from build123d import *

# Parameters (mm, degrees)
SKETCH10_R              = 10
BOSS_EXTRUDE1_DEPTH     = 5
CUT_EXTRUDE3_DEPTH      = 45
CUT_EXTRUDE3_DEPTH_BACK = 20
CUT_EXTRUDE5_DEPTH      = 5
BOSS_EXTRUDE2_DEPTH     = 5
SKETCH14_R              = 1
BOSS_EXTRUDE3_DEPTH     = 3
BOSS_EXTRUDE4_START     = 3
SKETCH15_R              = 1
BOSS_EXTRUDE4_DEPTH     = 3
CUT_EXTRUDE6_DEPTH      = 10
CUT_EXTRUDE6_DRAFT      = -10
SKETCH18_W              = 50.237541655
SKETCH18_H              = 20.454146011
CUT_EXTRUDE7_DEPTH      = 7
CUT_EXTRUDE7_DRAFT      = -30


with BuildPart() as part:
    # Sketch1 → Revolve1 (revolve)
    with BuildSketch(Plane.XY, mode=Mode.PRIVATE) as revolve1_sk:
        with BuildLine():
            Line((20.9, 0), (23.871591838, 0))
            Line((23.871591838, 0), (23.871591838, 4))
            Line((23.871591838, 4), (22.9, 4.236662843))
            Line((22.9, 4.236662843), (22.9, 11.874576818))
            ThreePointArc((22.9, 11.874576818), (23.83692213, 16.100759435), (26.472123903, 19.535021249))
            Line((26.472123903, 19.535021249), (26.427876097, 19.497892931))
            ThreePointArc((26.427876097, 19.497892931), (29.06307787, 22.932154745), (30, 27.158337362))
            Line((30, 27.158337362), (30, 50))
            ThreePointArc((30, 50), (28.828427125, 52.828427125), (26, 54))
            Line((26, 54), (0, 54))
            Line((0, 54), (0, 15))
            Line((0, 15), (19.9, 15))
            ThreePointArc((19.9, 15), (20.607106781, 14.707106781), (20.9, 14))
            Line((20.9, 14), (20.9, 0))
        make_face()
    revolve(revolve1_sk.sketch.rotate(Axis((0, 0, 0), (0, 1, 0)), 90), axis=Axis((0, 0, 0), (0, 1, 0)))

    # Sketch10 → Boss-Extrude1 (add)
    with BuildSketch(Plane(origin=(0, 0, -30), x_dir=(-1, 0, 0), z_dir=(0, 0, -1))):
        with Locations((3.346345887, 38.658337362)):
            Circle(SKETCH10_R)
    extrude(amount=-BOSS_EXTRUDE1_DEPTH)

    # Sketch11 → Cut-Extrude3 (cut, two sides: drawn at the far end of the back side and taken through both)
    with BuildSketch(Plane(origin=(0, 17, 0), x_dir=(1, 0, 0), z_dir=(0, 1, 0)).offset(-CUT_EXTRUDE3_DEPTH_BACK)):
        with BuildLine():
            Line((-17.5, 0), (17.5, 0))
            ThreePointArc((17.5, 0), (0, 17.5), (-17.5, 0))
        make_face()
    extrude(amount=CUT_EXTRUDE3_DEPTH + CUT_EXTRUDE3_DEPTH_BACK, mode=Mode.SUBTRACT)

    # Sketch9 → Cut-Extrude5 (cut)
    with BuildSketch(Plane(origin=(0, 54, 0), x_dir=(1, 0, 0), z_dir=(0, 1, 0))):
        with BuildLine():
            Line((-30, 0), (30, 0))
            ThreePointArc((30, 0), (0, 30), (-30, 0))
        make_face()
    extrude(amount=-CUT_EXTRUDE5_DEPTH, mode=Mode.SUBTRACT)

    # Sketch13 → Boss-Extrude2 (add)
    with BuildSketch(Plane(origin=(0, 0, 0), x_dir=(-1, 0, 0), z_dir=(0, 0, -1))):
        with BuildLine():
            Line((22.5, 53.5), (26.5, 53.5))
            ThreePointArc((26.5, 53.5), (26.853553391, 53.353553391), (27, 53))
            Line((27, 53), (27, 51))
            ThreePointArc((27, 51), (26.853553391, 50.646446609), (26.5, 50.5))
            Line((26.5, 50.5), (22.5, 50.5))
            ThreePointArc((22.5, 50.5), (22.146446609, 50.646446609), (22, 51))
            Line((22, 51), (22, 53))
            ThreePointArc((22, 53), (22.146446609, 53.353553391), (22.5, 53.5))
        make_face()
        with BuildLine():
            Line((-26.5, 53.5), (-22.5, 53.5))
            ThreePointArc((-22.5, 53.5), (-22.146446609, 53.353553391), (-22, 53))
            Line((-22, 53), (-22, 51))
            ThreePointArc((-22, 51), (-22.146446609, 50.646446609), (-22.5, 50.5))
            Line((-22.5, 50.5), (-26.5, 50.5))
            ThreePointArc((-26.5, 50.5), (-26.853553391, 50.646446609), (-27, 51))
            Line((-27, 51), (-27, 53))
            ThreePointArc((-27, 53), (-26.853553391, 53.353553391), (-26.5, 53.5))
        make_face()
    extrude(amount=BOSS_EXTRUDE2_DEPTH)

    # Sketch14 → Boss-Extrude3 (add)
    with BuildSketch(Plane.ZY.offset(-22)):
        with Locations(Location((-3, 52, 0), (0, 0, 270))):
            Circle(SKETCH14_R)
    extrude(amount=BOSS_EXTRUDE3_DEPTH)

    # Sketch15 → Boss-Extrude4 (add)
    with BuildSketch(Plane(origin=(-22, 0, 0), x_dir=(0, 0, -1), z_dir=(1, 0, 0)).offset(BOSS_EXTRUDE4_START)):
        with Locations(Location((3, 52, 0), (0, 0, 270))):
            Circle(SKETCH15_R)
    extrude(amount=-BOSS_EXTRUDE4_DEPTH)


with BuildPart() as cut_extrude6_tool:
    # Sketch17 → Cut-Extrude6 (with draft: the straight prism first)
    with BuildSketch(Plane(origin=(0, 0, 0), x_dir=(-1, 0, 0), z_dir=(0, 0, -1))):
        with BuildLine():
            ThreePointArc((-24.47851765, 47.302362136), (-25.892731213, 46.716575698), (-26.47851765, 45.302362136))
            Line((-26.47851765, 45.302362136), (-26.47851765, 25.01560965))
            ThreePointArc((-26.47851765, 25.01560965), (-25.892731213, 23.601396087), (-24.47851765, 23.01560965))
            Line((-24.47851765, 23.01560965), (25.354900287, 23.01560965))
            ThreePointArc((25.354900287, 23.01560965), (26.769113849, 23.601396087), (27.354900287, 25.01560965))
            Line((27.354900287, 25.01560965), (27.354900287, 45.302362136))
            ThreePointArc((27.354900287, 45.302362136), (26.769113849, 46.716575698), (25.354900287, 47.302362136))
            Line((25.354900287, 47.302362136), (-24.47851765, 47.302362136))
        make_face()
    extrude(amount=-CUT_EXTRUDE6_DEPTH)
    # Cut-Extrude6: the draft: its side faces are tilted about the plane it starts from
    cut_extrude6_sides = [cut_extrude6_tool.faces().sort_by_distance(p)[0] for p in [
        (25.892731213, 46.716575698, 5),
        (26.47851765, 35.158985893, 5),
        (25.892731213, 23.601396087, 5),
        (-0.438191318, 23.01560965, 5),
        (-26.769113849, 23.601396087, 5),
        (-27.354900287, 35.158985893, 5),
        (-26.769113849, 46.716575698, 5),
        (-0.438191318, 47.302362136, 5),
    ]]
    draft(cut_extrude6_sides, Plane(origin=(0, 0, 0), x_dir=(-1, 0, 0), z_dir=(0, 0, -1)), CUT_EXTRUDE6_DRAFT)


with BuildPart() as part_1:
    add(part.part)

    # Cut-Extrude6: cut by cut_extrude6_tool
    add(cut_extrude6_tool.part, mode=Mode.SUBTRACT)


with BuildPart() as cut_extrude7_tool:
    # Sketch18 → Cut-Extrude7 (with draft: the straight prism first)
    with BuildSketch(Plane(origin=(0, 0, 10), x_dir=(-1, 0, 0), z_dir=(0, 0, -1))):
        with Locations((0.403522985, 35.07528913)):
            Rectangle(SKETCH18_W, SKETCH18_H)
    extrude(amount=-CUT_EXTRUDE7_DEPTH)
    # Cut-Extrude7: the draft: its side faces are tilted about the plane it starts from
    cut_extrude7_sides = [cut_extrude7_tool.faces().sort_by_distance(p)[0] for p in [
        (24.715247843, 35.07528913, 13.5),
        (-0.403522984, 24.848216125, 13.5),
        (-25.522293812, 35.07528913, 13.5),
        (-0.403522984, 45.302362136, 13.5),
    ]]
    draft(cut_extrude7_sides, Plane(origin=(0, 0, 10), x_dir=(-1, 0, 0), z_dir=(0, 0, -1)), CUT_EXTRUDE7_DRAFT)


with BuildPart() as part_2:
    add(part_1.part)

    # Cut-Extrude7: cut by cut_extrude7_tool
    add(cut_extrude7_tool.part, mode=Mode.SUBTRACT)


solid = part_2.part
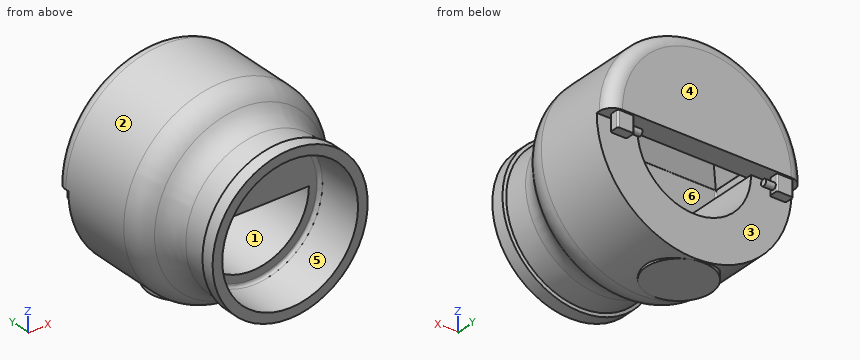
Geometry: final body of the model. Coordinates: model frame, mm. Face numbers are marked on the shaded views. A direction names the side the tool comes from. Round coordinates to 2 decimals unless told otherwise and drop trailing zeros. Loops run counter-clockwise (first coordinate to the right, second up) from the corner with the lowest first, then second, coordinate; pieces in that order, holes last. Notation, with made-up numbers: (36, 49.5) - (83, 49.5) arc R19 ccw to (83, 69.5) - close; hole circle Ø3 at (50, 1). An arc over 180 degrees is marked (long way). Write each question's results on one line, items separated by ' | '. Start each with the question number.
1) Mould query, pull axis X, two halves, no side actions, for the marked faces 1, 2 and 3. Classes: released by +X, released by -X, zero draft, split by the parting line, or undercut.
2) First-contact query: P1, Ø0.9, axis at x = -23.5, y = 52, coming from the -Z side; P2, Ø2, axis at y = 52, z = -1.5, coming from the -X side; P3, Ø1, axis at y = 52, z = -3.5, coming from the +X side. Flat tips, straight axial feed; report the tip coordinate or a pass-through.
3) Access query for the marked faces 4, 5 and 6. Directions: +Z, -Z, +X, -X, +Y, -Y. A direction counts if a zero-diameter tool reaches every point of the face in a straight line with its end or side. Return the directions, or none.
4) Line query: probe 1 along X at (y, z) = (10.25, 0); probe 2 along Y at (x, z) = (14, 4); probe 3 along Z at (x, y) = (-9, 22). Output: solid intervals per line, ascending. Write a range as [from, to].
5) Cut plane A-A on y = 52. Return loops of the section in (x, z).
6) Cut plane B-B on y = 18.5. Return loops of the section in (x, z), then the cut area to 3 significant figures.
Verdict:
1) face 1: undercut | face 2: split by the parting line | face 3: zero draft
2) P1: stops at z = -5 | P2: stops at x = -27 | P3: stops at x = 27
3) face 4: +Z, -Z, +X, -X, +Y | face 5: -Y | face 6: none
4) probe 1: x = [-22.9, -20.9], [20.9, 22.9] | probe 2: y = [15, 23.72], [46.6, 54] | probe 3: z = [-27.11, -15.01], [0, 27.11]
5) outline: (-29.46, 0) - (-27, 0) - (-27, -5) - (-22, -5) - (-22, -4) - (-19, -4) - (-19, -2) - (-22, -2) - (-22, 0) - (22, 0) - (22, -2) - (19, -2) - (19, -4) - (22, -4) - (22, -5) - (27, -5) - (27, 0) - (29.46, 0) arc R29.46 ccw to start
6) outline: circle Ø50.82 at (0, 0); hole (-17.5, 0) arc R17.5 ccw to (17.5, 0) - close | area: 1,550 mm2
